CAD build for the part. Positions are in the model's coordinates, mm. Round coordinates to 2 decimals unless told otherwise and drop trailing zeros. Loops run counter-clockwise (first coordinate to the right, second up) from the corner with the lowest first, then second, coordinate; pieces in that order, holes last. Notation, with made-up numbers: (39.25, 42.25) - (98.25, 42.25) arc R30 ccw to (98.25, 80.25) - close; hole circle Ø8 at (72.5, 79). An arc over 180 degrees is marked (long way). One line per question, with ' | ' between items.
Solid Edge part; units mm, degrees
sketch "Sketch1" plane through (0, 0, 0) normal (0, 0, 1) x (1, 0, 0)
  line L0 (0, 32) -> (7, 32)
  line L1 (7, 32) -> (7, 28)
  line L2 (7, 28) -> (5, 28)
  line L3 (2, 28) -> (5, 28)
  line L4 (0, 28) -> (2, 28)
  line L5 (0, 32) -> (0, 28)
  line L6 (0, 20) -> (7, 20)
  line L7 (7, 20) -> (7, 24)
  line L8 (7, 24) -> (5, 24)
  line L9 (2, 24) -> (5, 24)
  line L10 (0, 24) -> (2, 24)
  line L11 (0, 20) -> (0, 24)
  circle A0 centre (3.5, 26) radius 2.5
  dimension "D1" = 7
  dimension "D2" = 7
  dimension "D3" = 7
  dimension "D4" = 7
revolve "RevolvedProtrusion1" add sketch "Sketch1" angle 360 about axis through (0, 0, 0) along (1, 0, 0)
properties material "Aluminum, 6061-T6"
(1) Cut at A-A, the plane z = 0. Write the cut outline in (x, y).
Results found:
outline: (0, -32) - (7, -32) - (7, -28) - (5, -28) arc R2.5 ccw to (5, -24) - (7, -24) - (7, -20) - (0, -20) - (0, -24) - (2, -24) arc R2.5 ccw to (2, -28) - (0, -28) - close; (0, 20) - (7, 20) - (7, 24) - (5, 24) arc R2.5 ccw to (5, 28) - (7, 28) - (7, 32) - (0, 32) - (0, 28) - (2, 28) arc R2.5 ccw to (2, 24) - (0, 24) - close
(2) Two-plate mould, pull along Y, no slides. Class faces 1 (the face through (0, -0.1, -28.3)), 2 (the face through (3.55, -6.94, -31.24)), 3 (the face through (5.986, -23.977, -1.055)): released by +Y, released by -Y, zero draft, split by the parting line, or undercut.
Results found:
face 1: zero draft | face 2: split by the parting line | face 3: undercut
(3) Drop flat-ended pins along their axis: P1, Ø3, axis at x = 3, z = 12, coming from the +Y side; P2, Ø3, axis at x = 1, y = -17.5, coming from the +Z side; P3, Ø1.5, axis at x = 3, y = 0.5, coming from the +Z side. Give the stop position or say it passes through.
Results found:
P1: stops at y = 30.23 | P2: stops at z = 27.71 | P3: stops at z = 32
(4) Probe L1, parallel to Z at x = 6.1, y = 0; L2, parallel to Y at x = 5.5, z = -5.5; L3, parallel to Z at x = 6.25, y = -9.5. List the from-to ranges inside material, lowest first.
Results found:
L1: z = -32 to -28, -24 to -20, 20 to 24, 28 to 32 | L2: y = -31.52 to -27.45, -26.94 to -23.87, -23.36 to -19.23, 19.23 to 23.36, 23.87 to 26.94, 27.45 to 31.52 | L3: z = -30.56 to -26.34, -22.04 to -17.6, 17.6 to 22.04, 26.34 to 30.56
